Solid Edge part; units mm, degrees
sketch "Sketch1" plane through (0, 0, 0) normal (0, 0, 1) x (1, 0, 0)
  circle A0 centre (0, 0) radius 1.5
  circle A1 centre (0, 0) radius 5
extrude "Protrusion1" add sketch "Sketch1" along normal mid plane 4
sketch "Sketch2" plane through (0, 0, 0) normal (0, -1, 0) x (1, 0, 0)
  line L0 (0, 2) -> (2.5, 2)
  line L1 (2.5, 2) -> (2.5, 1.6)
  line L2 (2.5, 1.6) -> (4.5, 1.6)
  line L3 (4.5, 1.6) -> (4.5, 2)
  line L4 (4.5, 2) -> (5.6166, 2)
  dimension "D1" = 4.5
  dimension "D2" = 2.5
revolve "RevolvedCutout1" cut sketch "Sketch2" angle 360 about axis through (0, 0, 54) along (0, 0, -1) material side at (1.25, 0, 2.05)
mirror "Mirror1" about plane through (0, 0, 0) normal (0, 0, 1) of "RevolvedCutout1"
properties material "Stainless steel"
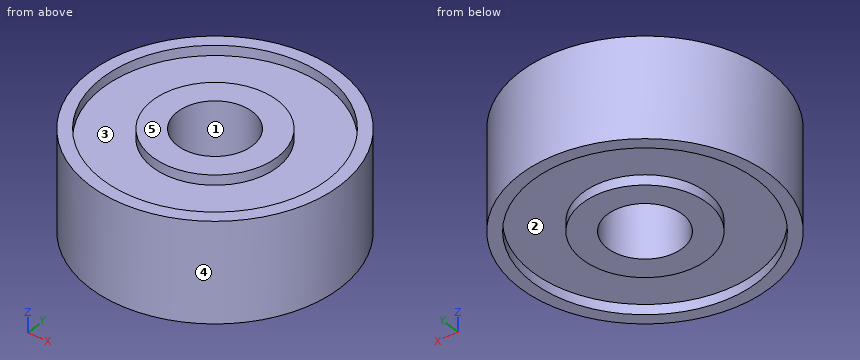
Input: part model. Units: mm. Frame: model coordinates. Face numbers are marked on the shaded views. A direction names the side the tool comes from. Coordinates: 2 decimals unless noted, no trailing zeros. Loops run counter-clockwise (first coordinate to the right, second up) from the corner with the lowest first, then second, coordinate; pieces in that order, holes last. Notation, with made-up numbers: M 19.5,29 L 51.5,29 A27 ccw 51.5,63 Z; hole C 55.25,17.5 d2. An arc over 180 degrees is marked long. Answer in a Markdown table with one row per item.
1. Material intervals for line 1 (Y direction, x = 0, z = 1.95); line 2 (Y direction, x = 0, z = 0.15); line 3 (Y direction, x = -2.25, z = -1.8), sorted ascending.
Response:
| item | result |
|---|---|
| line 1 | y = -5 to -4.5, -2.5 to -1.5, 1.5 to 2.5, 4.5 to 5 |
| line 2 | y = -5 to -1.5, 1.5 to 5 |
| line 3 | y = -4.47 to -3.9, -1.09 to 1.09, 3.9 to 4.47 |
2. Draft query along Y for the marked faces 3, 4 and 5. Return one class per face: pulls with the +Y half, pulls with the -Y half, needs draft (parallel to the pull), parting line crosses it, or undercut.
Response:
| item | result |
|---|---|
| face 3 | undercut |
| face 4 | parting line crosses it |
| face 5 | needs draft |
3. Section C-C, the plane z = -0.4. Output: boundary loops of the cut face in (x, y), then the cut area to 3 significant figures.
Response:
| item | result |
|---|---|
| outline | C 0,0 d10; hole C 0,0 d3 |
| area | 71.5 mm2 |
4. Section A-A, the plane y = 0. Output: boundary loops of the cut face in (x, z).
Response:
| item | result |
|---|---|
| outline | M -5,-2 L -4.5,-2 L -4.5,-1.6 L -2.5,-1.6 L -2.5,-2 L -1.5,-2 L -1.5,2 L -2.5,2 L -2.5,1.6 L -4.5,1.6 L -4.5,2 L -5,2 Z; M 1.5,-2 L 2.5,-2 L 2.5,-1.6 L 4.5,-1.6 L 4.5,-2 L 5,-2 L 5,2 L 4.5,2 L 4.5,1.6 L 2.5,1.6 L 2.5,2 L 1.5,2 Z |
5. First-contact query: pin 1 (1 mm diameter, centred on y = -2.5, z = -1, fed in from -X); pin 2 (2.5 mm diameter, centred on x = 0, y = 0, fed in from +Z); pin 3 (1.5 mm diameter, centred on y = 2, z = -1, fed in from +X); pin 4 (1.5 mm diameter, centred on x = 1.5, z = 1.5, fed in from -Y). Flat tips, straight axial feed; report the tip coordinate or a pass-through.
Response:
| item | result |
|---|---|
| pin 1 | stops at x = -4.58 |
| pin 2 | passes through |
| pin 3 | stops at x = 4.84 |
| pin 4 | stops at y = -4.94 |
6. Section D-D, the plane x = -4. Output: boundary loops of the cut face in (y, z), then the cut area to 3 significant figures.
Response:
| item | result |
|---|---|
| outline | M -3,-2 L -2.06,-2 L -2.06,-1.6 L 2.06,-1.6 L 2.06,-2 L 3,-2 L 3,2 L 2.06,2 L 2.06,1.6 L -2.06,1.6 L -2.06,2 L -3,2 Z |
| area | 20.7 mm2 |
7. Reachability of the marked faces 1 and 2 from +Z, -Z, +X, -X, +Y, -Y: full face, straight path, thin tool, end or side. Return the list, or none.
Response:
| item | result |
|---|---|
| face 1 | +Z, -Z |
| face 2 | -Z |
